```python
from build123d import *

# Parameters (mm, degrees)
SKETCH1_W           = 40
SKETCH1_H           = 40
BOSS_EXTRUDE1_DEPTH = 10
SKETCH2_W           = 6
SKETCH2_H           = 6
CUT_EXTRUDE1_DEPTH  = 5
SKETCH3_W           = 6
SKETCH3_H           = 6
BOSS_EXTRUDE2_DEPTH = 5


with BuildPart() as part:
    # Sketch1 → Boss-Extrude1 (new body)
    with BuildSketch(Plane.XY):
        with Locations((0, 20)):
            Rectangle(SKETCH1_W, SKETCH1_H)
    extrude(amount=BOSS_EXTRUDE1_DEPTH)

    # Sketch2 → Cut-Extrude1 (cut)
    with BuildSketch(Plane.XY):
        with Locations((-11, 11)):
            Rectangle(SKETCH2_W, SKETCH2_H)
    cut_extrude1 = extrude(amount=CUT_EXTRUDE1_DEPTH, mode=Mode.SUBTRACT)

    # Sketch3 → Boss-Extrude2 (add)
    with BuildSketch(Plane.XY.offset(10)):
        with Locations((-11, 27)):
            Rectangle(SKETCH3_W, SKETCH3_H)
    boss_extrude2 = extrude(amount=BOSS_EXTRUDE2_DEPTH)

    # Mirror1: Cut-Extrude1, Boss-Extrude2 across plane
    add(cut_extrude1.mirror(Plane(origin=(0, 0, 0), x_dir=(0, 0, 1), z_dir=(1, 0, 0))), mode=Mode.SUBTRACT)
    add(boss_extrude2.mirror(Plane(origin=(0, 0, 0), x_dir=(0, 0, 1), z_dir=(1, 0, 0))))


solid = part.part
```
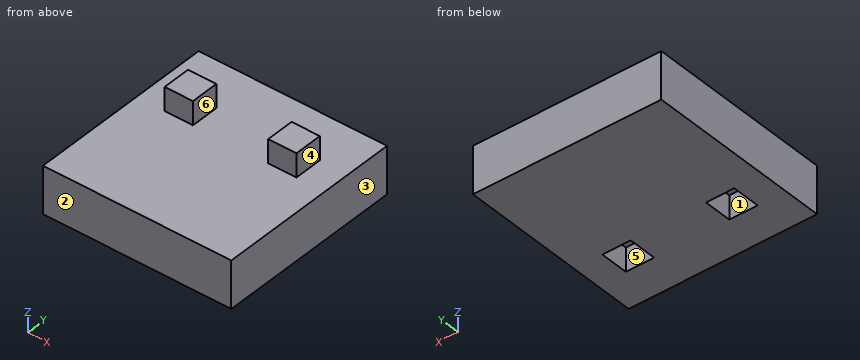
Geometry: final body of the model. Coordinates: model frame, mm. Face numbers are marked on the shaded views. A direction names the side the tool comes from. Round coordinates to 2 decimals unless told otherwise and drop trailing zeros. Order: outer loops, then holes, each group sorted by start corner. A loop starts at its lowest first (then second) coordinate and runs counter-clockwise, first axis right, second up. Notation, with made-up numbers: (-15, 21) -> (11, 21) arc R17 cw to (11, 44) -> close; hole circle Ø8 at (6, 58.5). An arc over 180 degrees is marked (long way). Use one line per item in the form item = value.
(1) Access query for the marked faces 4, 5 and 6. Directions: +Z, -Z, +X, -X, +Y, -Y. A direction counts if a zero-diameter tool reaches every point of the face in a straight line with its end or side. Return the directions, or none.
Results list:
face_4 = +Z, +X, +Y, -Y
face_5 = -Z
face_6 = +Z, +Y, -Y
(2) Ray query, probe 1 along Y at (x, z) = (-10.5, 2.5); probe 2 along Z at (x, y) = (6.5, 24.5); probe 3 along Y at (x, z) = (13, 14). Return the intervals inside material, ascending. Write a range as [from, to].
Results list:
probe_1 = [0, 8], [14, 40]
probe_2 = [0, 10]
probe_3 = [24, 30]
(3) Section D-D on y = 29. Return loops of the section in (x, z).
Results list:
outline = (-20, 0) -> (20, 0) -> (20, 10) -> (14, 10) -> (14, 15) -> (8, 15) -> (8, 10) -> (-8, 10) -> (-8, 15) -> (-14, 15) -> (-14, 10) -> (-20, 10) -> close
(4) Section B-B on z = 3. Return loops of the section in (x, y), and give its area (3 significant figures).
Results list:
outline = (-20, 0) -> (20, 0) -> (20, 40) -> (-20, 40) -> close; hole (-14, 8) -> (-8, 8) -> (-8, 14) -> (-14, 14) -> close; hole (8, 8) -> (14, 8) -> (14, 14) -> (8, 14) -> close
area = 1,530 mm^2
(5) Draft query along X for the marked faces 1, 2 and 3. Return one class per face: pulls with the +X half, pulls with the -X half, needs draft (parallel to the pull), parting line crosses it, or undercut.
Results list:
face_1 = undercut
face_2 = needs draft
face_3 = pulls with the +X half
(6) Section A-A on z = 12.5. Return loops of the section in (x, y).
Results list:
outline = (-14, 24) -> (-8, 24) -> (-8, 30) -> (-14, 30) -> close; (8, 24) -> (14, 24) -> (14, 30) -> (8, 30) -> close
(7) Section C-C on x = -9.5. Return loops of the section in (y, z).
Results list:
outline = (0, 0) -> (8, 0) -> (8, 5) -> (14, 5) -> (14, 0) -> (40, 0) -> (40, 10) -> (30, 10) -> (30, 15) -> (24, 15) -> (24, 10) -> (0, 10) -> close
(8) First-contact query: pin 1 Ø1 at (x, y) = (-7.5, 19.5) entering from +Z; pin 2 Ø4 at (y, z) = (27.5, 13.5) entering from -X; pin 3 Ø2.5 at (x, z) = (-12, 13.5) entering from -Y. Flat tips, straight axial feed; report the tip coordinate or a pass-through.
Results list:
pin_1 = 10
pin_2 = -14
pin_3 = 24
